Verification items for this drawing (mm, ordinates from the low corner). Round coordinates to 2 decimals unless told otherwise and drop trailing zeros. Order: outer loops, then holes, each group sorted by start corner. A loop starts at its lowest first (then second) coordinate and runs counter-clockwise, first axis right, second up. Notation, with made-up numbers: M -1,68.5 L 20,68.5 A23 ccw 20,100.5 Z; hole C -37,87 d4. An arc over 180 degrees is marked long. Return JSON: item names as keys, results as strings. Group by question number.
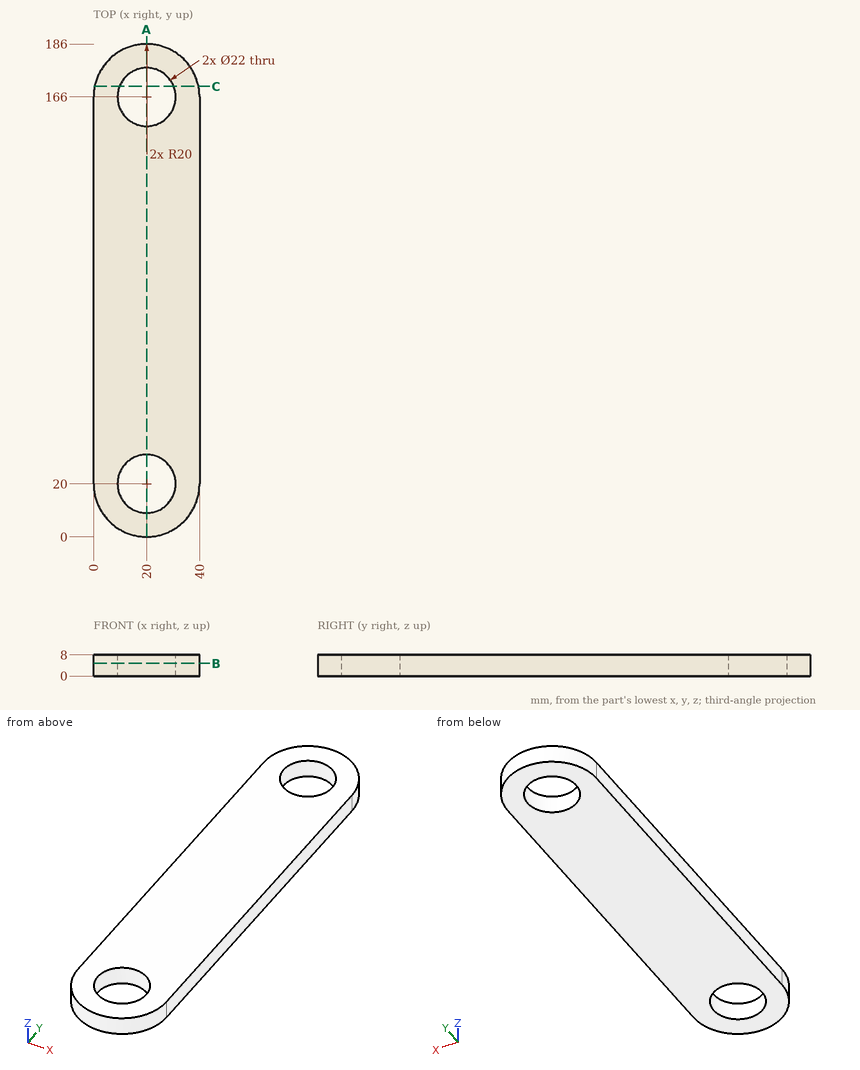
1. Cross-section at B-B (z = 4.75). Enter the section's corners in (x, y).
2. Cross-section at A-A (x = 20). Enter the section's corners in (y, z), plus the area to 3 significant figures.
3. Cross-section at C-C (y = 170). Enter the section's corners in (x, z), plus the area to 3 significant figures.
4. Thickness scan on line 1 along Y through (x, z) = (20, 6.25); line 2 along X through (y, z) = (165.5, 5.25); line 3 along Y through (x, z) = (22, 3). Record the ranges inside material, lowest first. Write a range as from..to.
5. Go/stop test with flat-tipped pins: pin 1 (2 mm diameter, centred on x = 10, z = 1, fed in from +Y); pin 2 (1 mm diameter, centred on x = 14.5, z = 2, fed in from -Y); pin 3 (1 mm diameter, centred on x = 32.5, z = 2.5, fed in from -Y). Record where each tip stops, or that it passes through.
Computed:
{
 "1": {"outline": "M 0,20 A20 ccw 40,20 L 40,166 A20 ccw 0,166 Z; hole C 20,20 d22; hole C 20,166 d22"},
 "2": {"outline": "M 0,0 L 9,0 L 9,8 L 0,8 Z; M 31,0 L 155,0 L 155,8 L 31,8 Z; M 177,0 L 186,0 L 186,8 L 177,8 Z", "area": "1,140 mm²"},
 "3": {"outline": "M 0.4,0 L 9.75,0 L 9.75,8 L 0.4,8 Z; M 30.25,0 L 39.6,0 L 39.6,8 L 30.25,8 Z", "area": "150 mm²"},
 "4": {"line 1": "y = 0..9, 31..155, 177..186", "line 2": "x = 0..9.01, 30.99..40", "line 3": "y = 0.1..9.18, 30.82..155.18, 176.82..185.9"},
 "5": {"pin 1": "stops at y = 183.86", "pin 2": "stops at y = 0.64", "pin 3": "stops at y = 4"}
}
